```python
from build123d import *

# Parameters (mm, degrees)
SKETCH_1_R          = 11
EXTRUDE_1_DEPTH     = 5
SKETCH_2_R          = 3.25
EXTRUDE_2_DEPTH     = 20
FILLET_1_R          = 1
EXTRUDE_3_DEPTH     = 5
FILLET_2_R          = 2
SKETCH_4_R          = 1.6
CUT_EXTRUDE_1_DEPTH = 5


with BuildPart() as part:
    # 草图1 → 凸台-拉伸1 (new body)
    with BuildSketch(Plane.XY):
        with BuildLine():
            Line((-4.49108361, 30.19776432), (-27.49108361, -16.80223568))
            ThreePointArc((-27.49108361, -16.80223568), (-27.241981942, -21.64680736), (-23, -24))
            Line((-23, -24), (23, -24))
            ThreePointArc((23, -24), (27.241981942, -21.64680736), (27.49108361, -16.80223568))
            Line((27.49108361, -16.80223568), (4.49108361, 30.19776432))
            ThreePointArc((4.49108361, 30.19776432), (0, 33), (-4.49108361, 30.19776432))
        make_face()
        Circle(SKETCH_1_R, mode=Mode.SUBTRACT)
    extrude(amount=EXTRUDE_1_DEPTH)

    # 草图2 → 凸台-拉伸2 (add)
    with BuildSketch(Plane(origin=(0, 0, 0), x_dir=(-1, 0, 0), z_dir=(0, 0, -1))):
        with Locations(Location((0, 28, 0), (0, 0, 180))):
            Circle(SKETCH_2_R)
        with Locations(Location((-23, -19, 0), (0, 0, 180))):
            Circle(SKETCH_2_R)
        with Locations(Location((23, -19, 0), (0, 0, 180))):
            Circle(SKETCH_2_R)
    extrude(amount=EXTRUDE_2_DEPTH)

    # 圆角1
    fillet_1_edges = [part.edges().sort_by_distance(p)[0] for p in [
        (-3.25, 28, 0),
        (19.75, -19, 0),
        (-26.25, -19, 0),
    ]]
    fillet(fillet_1_edges, radius=FILLET_1_R)

    # 草图3 → 凸台-拉伸3 (add)
    with BuildSketch(Plane.XY.offset(5)):
        Polygon((-20, 20), (-9.481478916, 20), (-20, -1.494369172), align=None)
        Polygon((20, 20), (20, -1.494369172), (9.481478916, 20), align=None)
    extrude(amount=-EXTRUDE_3_DEPTH)

    # 圆角2
    fillet_2_edges = [part.edges().sort_by_distance(p)[0] for p in [
        (-20, -1.494369172, 2.5),
        (-20, 20, 2.5),
        (20, 20, 2.5),
        (20, -1.494369172, 2.5),
    ]]
    fillet(fillet_2_edges, radius=FILLET_2_R)

    # 草图4 → 切除-拉伸1 (cut)
    with BuildSketch(Plane.XY.offset(5)):
        with Locations((-15, 15)):
            Circle(SKETCH_4_R)
        with Locations((15, 15)):
            Circle(SKETCH_4_R)
        with Locations((15, -3)):
            Circle(SKETCH_4_R)
        with Locations((-15, -3)):
            Circle(SKETCH_4_R)
    extrude(amount=-CUT_EXTRUDE_1_DEPTH, mode=Mode.SUBTRACT)


solid = part.part
```
Model file for the job. Use its own axes, mm. A direction names the side the tool comes from. Give positions to 0.01 mm unless a question says otherwise; leave off trailing zeros. Order: outer loops, then holes, each group sorted by start corner. A loop starts at its lowest first (then second) coordinate and runs counter-clockwise, first axis right, second up.
1) Pin check, flat tips, straight feed: pin 1 (3.5 mm diameter, centred on x = -15, y = -3, fed in from -Z); pin 2 (1 mm diameter, centred on x = -2.5, z = -14, fed in from -Y); pin 3 (4 mm diameter, centred on x = 15.5, z = 1.5, fed in from +Y). Stop position of each tip, or through.
2) Saw through at A-A, the plane y = 0. Write the cut outline in (x, z), then the cut area to 3 significant figures.
3) Wall check: probe 1 along Y at (x, z) = (15, 3.5); probe 2 along Y at (x, z) = (0, 1.5); probe 3 along Z at (x, y) = (-7, 24.5). Give the ranges that are in metal, low to high.
4) Saw through at B-B, the plane x = 0. Write the cut outline in (y, z), then the cut area to 3 significant figures.
5) Saw through at C-C, the plane x = -15. Write the cut outline in (y, z), then the cut area to 3 significant figures.
6) 3-axis set-ups, long thin cutter, end or side, ignore diameter. For faces 1 (the flat face through (-14, 20, 3)), 2 (the cylindrical face through (-0.705, 31.173, -10.367)), 3 (the flat face through (20, 9, 3)): which of +Z, -Z, +X, -X, +Y, -Y reach the whole face in a straight line?
7) Mould opens along Y. For faces 4 (the flat face through (23, -19, -20)), 5 (the flat face through (0, -24, 2)), 6 (the cylindrical face through (-16.6, -2.93, 2.54)) say: +Y half, -Y half, draft (parallel to the pull), parting line (faces both ways), or undercut.
8) Saw through at D-D, the plane z = 2.5. Write the cut outline in (x, y), then the cut area to 3 significant figures.
Computed:
1. pin 1: stops at z = 0
1. pin 2: stops at y = 25.44
1. pin 3: stops at y = 20
2. outline: (-20, 0) - (-11, 0) - (-11, 5) - (-20, 5) - close; (11, 0) - (20, 0) - (20, 5) - (11, 5) - close
2. area: 90.0 mm2
3. probe 1: y = -24 to -4.6, -1.4 to 13.4, 16.6 to 20
3. probe 2: y = -24 to -11, 11 to 33
3. probe 3: z = 0 to 5
4. outline: (-24, 0) - (-11, 0) - (-11, 5) - (-24, 5) - close; (11, 0) - (23.75, 0) arc R1 cw to (24.75, -1) - (24.75, -20) - (31.25, -20) - (31.25, -1) arc R1 cw to (32.25, 0) - (33, 0) - (33, 5) - (11, 5) - close
4. area: 305 mm2
5. outline: (-24, 0) - (-4.6, 0) - (-4.6, 5) - (-24, 5) - close; (-1.4, 0) - (13.4, 0) - (13.4, 5) - (-1.4, 5) - close; (16.6, 0) - (20, 0) - (20, 5) - (16.6, 5) - close
5. area: 188 mm2
6. face 1: +Z, -Z, -X, +Y
6. face 2: -Z
6. face 3: +Z, -Z, +X, +Y
7. face 4: draft
7. face 5: -Y half
7. face 6: undercut
8. outline: (-27.49, -16.8) arc R5 ccw to (-23, -24) - (23, -24) arc R5 ccw to (27.49, -16.8) - (20.2, -1.91) arc R2 cw to (20, -1.03) - (20, 18) arc R2 ccw to (18, 20) - (9.48, 20) - (4.49, 30.2) arc R5 ccw to (-4.49, 30.2) - (-9.48, 20) - (-18, 20) arc R2 ccw to (-20, 18) - (-20, -1.03) arc R2 cw to (-20.2, -1.91) - close; hole circle Ø3.2 at (-15, -3); hole circle Ø3.2 at (-15, 15); hole circle Ø22 at (0, 0); hole circle Ø3.2 at (15, -3); hole circle Ø3.2 at (15, 15)
8. area: 1,720 mm2
